from build123d import *

# Parameters (mm, degrees)
SKETCH_1_R          = 3.4
EXTRUDE_1_DEPTH     = 3.2
SKETCH_1_3_R        = 3.4
EXTRUDE_2_DEPTH     = 5
SKETCH_2_R          = 2
CUT_EXTRUDE_1_DEPTH = 5


with BuildPart() as part:
    # Sketch 1 → Extrude 1 (new body)
    with BuildSketch(Plane(origin=(0, 0, 0), x_dir=(1, 0, 0), z_dir=(0, 1, 0))):
        with BuildLine():
            Line((2.788583706, -2.763536548), (3.288084146, -0.865160476))
            ThreePointArc((3.288084146, -0.865160476), (2.414984165, -2.39329302), (0.894791131, -3.280144636))
            Line((0.894791131, -3.280144636), (2.788583706, -2.763536548))
        make_face()
        with BuildLine():
            Line((3.288084146, -0.865160476), (3.787584707, 1.033216056))
            Line((3.787584707, 1.033216056), (2.39329268, 2.414984502))
            ThreePointArc((2.39329268, 2.414984502), (3.13824753, 1.308205811), (3.4, 0))
            ThreePointArc((3.4, 0), (3.371904958, -0.436184539), (3.288084146, -0.865160476))
        make_face()
        with BuildLine():
            ThreePointArc((-0.894791101, 3.280144644), (0.865160253, 3.288084205), (2.39329268, 2.414984502))
            Line((2.39329268, 2.414984502), (0.999001002, 3.796752603))
            Line((0.999001002, 3.796752603), (-0.894791101, 3.280144644))
        make_face()
        with BuildLine():
            ThreePointArc((-3.288084139, 0.865160504), (-2.414984144, 2.393293042), (-0.894791101, 3.280144644))
            Line((-0.894791101, 3.280144644), (-2.788583706, 2.763536548))
            Line((-2.788583706, 2.763536548), (-3.288084139, 0.865160504))
        make_face()
        with BuildLine():
            ThreePointArc((-2.393292658, -2.414984524), (-3.280144574, -0.894791357), (-3.288084139, 0.865160504))
            Line((-3.288084139, 0.865160504), (-3.787584707, -1.033216056))
            Line((-3.787584707, -1.033216056), (-2.393292658, -2.414984524))
        make_face()
        Circle(SKETCH_1_R)
        with BuildLine():
            Line((-0.999001002, -3.796752603), (0.894791131, -3.280144636))
            ThreePointArc((0.894791131, -3.280144636), (-0.865160223, -3.288084212), (-2.393292658, -2.414984524))
            Line((-2.393292658, -2.414984524), (-0.999001002, -3.796752603))
        make_face()
    extrude(amount=EXTRUDE_1_DEPTH)

    # Sketch 1_3 → Extrude 2 (add)
    with BuildSketch(Plane(origin=(0, 0, 0), x_dir=(1, 0, 0), z_dir=(0, 1, 0))):
        Circle(SKETCH_1_3_R)
    extrude(amount=EXTRUDE_2_DEPTH)

    # Sketch 2 → Cut-Extrude 1 (cut)
    with BuildSketch(Plane(origin=(0, 0, 0), x_dir=(1, 0, 0), z_dir=(0, 1, 0))):
        Circle(SKETCH_2_R)
    extrude(amount=CUT_EXTRUDE_1_DEPTH, mode=Mode.SUBTRACT)


solid = part.part
Geometry: final body of the model. Coordinates: model frame, mm. A direction names the side the tool comes from. Coordinates: 2 decimals unless noted, no trailing zeros. Loops run counter-clockwise (first coordinate to the right, second up) from the corner with the lowest first, then second, coordinate; pieces in that order, holes last. Notation, with made-up numbers: M 80,85 L 119,85 A9 cw 119,98 Z; hole C 78.25,87.25 d10. An arc over 180 degrees is marked long. One line per item, written item: value. Start each with the question number.
1) Cut plane D-D (x = -3). Return loops of the section in (y, z), then the cut area to 3 significant figures.
2) Cut plane B-B (z = 0). Return loops of the section in (x, y), then the cut area to 3 significant figures.
3) Cut plane A-A (y = 2.85). Return loops of the section in (x, z).
4) Material intervals for L1, parallel to Z at x = 0, y = 3.4; L2, parallel to Y at x = -1.5, z = 3.25, sorted ascending. Write a range as from..to.
5) Pin query (flat end, axial travel): P1, Ø3, axis at x = 2.5, y = 3.5, coming from the +Z side; P2, Ø1, axis at y = 1.5, z = -0.5, coming from the +X side; P3, Ø2.5, axis at x = 0, z = 0, coming from the +Y side. Return the tip coordinate at first contact, or that it passes through.
6) Cut plane C-C (x = 0). Return loops of the section in (y, z).
7) Reachability of faces 1 (the flat face through (0, 5, 2.2)), 2 (the flat face through (2.53, 3.2, 2.51)), 3 (the flat face through (-2.54, 3.2, -2.53)) from +Z, -Z, +X, -X, +Y, -Y: full face, straight path, thin tool, end or side. Return the list, or none.
8) Draft query along X for faces 4 (the cylindrical face through (-0.74, 4.09, 3.32)), 5 (the flat face through (2, 0, 2)), 6 (the cylindrical face through (0, 2, 2)). Return one class per face: released by +X, released by -X, zero draft, split by the parting line, or undercut.
Evaluation:
1. outline: M 0,-1.96 L 3.2,-1.96 L 3.2,-1.6 L 5,-1.6 L 5,1.6 L 3.2,1.6 L 3.2,1.81 L 0,1.81 Z
1. area: 17.8 mm^2
2. outline: M -3.52,0 L -2,0 L -2,5 L -3.4,5 L -3.4,3.2 L -3.52,3.2 Z; M 2,0 L 3.52,0 L 3.52,3.2 L 3.4,3.2 L 3.4,5 L 2,5 Z
2. area: 14.7 mm^2
3. outline: M -3.79,1.03 L -2.79,-2.76 L 1,-3.8 L 3.79,-1.03 L 2.79,2.76 L -1,3.8 Z; hole C 0,0 d4
4. L1: -3.4..-2, 2..3.4
4. L2: 0..3.2
5. P1: z = 3.25
5. P2: x = 3.78
5. P3: through
6. outline: M 0,-3.52 L 3.2,-3.52 L 3.2,-3.4 L 5,-3.4 L 5,-2 L 0,-2 Z; M 0,2 L 5,2 L 5,3.4 L 3.2,3.4 L 3.2,3.52 L 0,3.52 Z
7. face 1: +Z, -Z, +X, -X, +Y
7. face 2: +Z, +X, +Y
7. face 3: -Z, -X, +Y
8. face 4: split by the parting line
8. face 5: zero draft
8. face 6: undercut
